from build123d import *

# Parameters (mm, degrees)
BOSS_EXTRUDE1_DEPTH     = 40
SKETCH2_R               = 2.6
CUT_EXTRUDE1_DEPTH      = 40
CUT_EXTRUDE2_DEPTH      = 3
CUT_EXTRUDE3_DEPTH      = 52.23475383
CUT_EXTRUDE3_DEPTH_BACK = 52.23475383
SKETCH4_R               = 2.6
CUT_EXTRUDE4_DEPTH      = 3
CHAMFER1_SIZE           = 10


with BuildPart() as part:
    # Sketch1 → Boss-Extrude1 (new body)
    with BuildSketch(Plane(origin=(0, 0, 0), x_dir=(1, 0, 0), z_dir=(0, 1, 0))):
        Polygon((0, 0), (25, 0), (25, 5), (5, 5), (5, 25), (0, 25), align=None)
    extrude(amount=BOSS_EXTRUDE1_DEPTH)

    # Sketch2 → Cut-Extrude1 (cut)
    with BuildSketch(Plane(origin=(0, 0, -5), x_dir=(-1, 0, 0), z_dir=(0, 0, -1))):
        with Locations((-17, 20)):
            Circle(SKETCH2_R)
    extrude(amount=-CUT_EXTRUDE1_DEPTH, mode=Mode.SUBTRACT)

    # Sketch3 → Cut-Extrude2 (cut)
    with BuildSketch(Plane(origin=(0, 0, -5), x_dir=(-1, 0, 0), z_dir=(0, 0, -1))):
        Polygon((-14.546261356, 24.25), (-19.453738644, 24.25), (-21.907477288, 20), (-19.453738644, 15.75), (-14.546261356, 15.75), (-12.092522712, 20), align=None)
    extrude(amount=-CUT_EXTRUDE2_DEPTH, mode=Mode.SUBTRACT)

    # Sketch4 → Cut-Extrude3 (cut, two sides: drawn at the far end of the back side and taken through both)
    with BuildSketch(Plane(origin=(5, 0, 0), x_dir=(0, 0, -1), z_dir=(1, 0, 0)).offset(-CUT_EXTRUDE3_DEPTH_BACK)):
        with Locations((17, 20)):
            Circle(SKETCH4_R)
    extrude(amount=CUT_EXTRUDE3_DEPTH + CUT_EXTRUDE3_DEPTH_BACK, mode=Mode.SUBTRACT)

    # Sketch5 → Cut-Extrude4 (cut)
    with BuildSketch(Plane(origin=(5, 0, 0), x_dir=(0, 0, -1), z_dir=(1, 0, 0))):
        Polygon((19.453738644, 24.25), (14.546261356, 24.25), (12.092522712, 20), (14.546261356, 15.75), (19.453738644, 15.75), (21.907477288, 20), align=None)
    extrude(amount=-CUT_EXTRUDE4_DEPTH, mode=Mode.SUBTRACT)

    # Chamfer1
    chamfer1_edges = [part.edges().sort_by_distance(p)[0] for p in [
        (25, 40, -2.5),
        (2.5, 40, -25),
        (2.5, 0, -25),
        (25, 0, -2.5),
    ]]
    chamfer(chamfer1_edges, length=CHAMFER1_SIZE)


solid = part.part
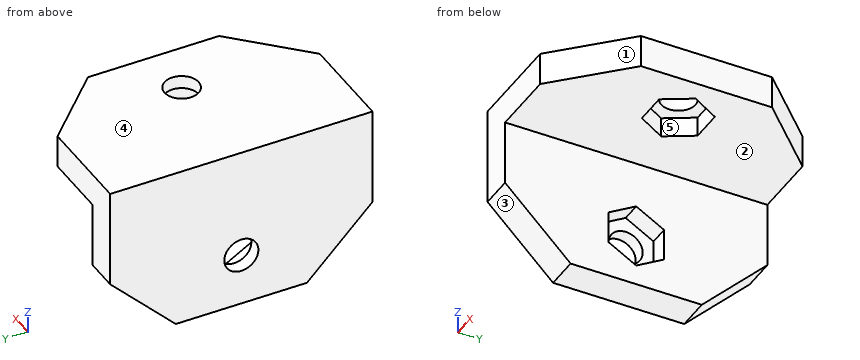
Verification items for the finished model (mm, model axes). Face numbers are marked on the shaded views. A direction names the side the tool comes from. Coordinates: 2 decimals unless noted, no trailing zeros. Order: outer loops, then holes, each group sorted by start corner. A loop starts at its lowest first (then second) coordinate and runs counter-clockwise, first axis right, second up. Notation, with made-up numbers: (87, -18.5) -> (141, -18.5) arc R18 ccw to (141, -8.5) -> close; hole circle Ø4 at (-10, -32.5). An arc over 180 degrees is marked (long way). Put each result on its own line as item: value. Start each with the question number.
1. Mould release check, pull along Y, two halves, no side actions. Record for the marked faces 3, 4 and 5: released by +Y, released by -Y, zero draft, split by the parting line, or undercut.
2. Access from +Z, -Z, +X, -X, +Y, -Y to the whole of each face (thin tool, end or side, straight path). Record for the marked faces 1 and 2.
3. Cross-section at A-A, the plane x = 17. Record the boundary of the cut face in (y, z), then the cut area to 3 significant figures.
4. Cross-section at D-D, the plane z = -13.75. Record the boundary of the cut face in (x, y), then the cut area to 3 significant figures.
5. Cross-section at C-C, the plane y = 18.5. Record the boundary of the cut face in (x, z).
6. Cross-section at B-B, the plane z = -17. Record the boundary of the cut face in (x, y).
7. Go/stop test with flat-tipped pins: pin 1 Ø12 at (x, z) = (13, -11.5) entering from -Y; pin 2 Ø3 at (x, y) = (10.5, 7) entering from -Z; pin 3 Ø2.5 at (x, z) = (4, -18) entering from +Y; pin 4 Ø2.5 at (x, z) = (16.5, -3) entering from -Y. Record where each tip stops, or that it passes through.
8. Material ranges on L1, parallel to Z at x = 1, y = 20; L2, parallel to Y at x = 2.5, z = -14.75; L3, parallel to X at y = 9, z = -10.25, recorded low to high. Write a range as [from, to].
Computed:
1. face 3: released by -Y
1. face 4: zero draft
1. face 5: undercut
2. face 1: +Z, -Z, +X, -Y
2. face 2: -Z, +X, +Y, -Y
3. outline: (2, -5) -> (15.75, -5) -> (15.75, -2) -> (17.4, -2) -> (17.4, 0) -> (2, 0) -> close; (22.6, -2) -> (24.25, -2) -> (24.25, -5) -> (38, -5) -> (38, 0) -> (22.6, 0) -> close
3. area: 144 mm2
4. outline: (0, 0) -> (5, 0) -> (5, 17.13) -> (2, 17.13) -> (2, 22.87) -> (5, 22.87) -> (5, 40) -> (0, 40) -> close
4. area: 183 mm2
5. outline: (0, -25) -> (5, -25) -> (5, -21.04) -> (2, -21.04) -> (2, -19.12) -> (0, -19.12) -> close; (0, -14.88) -> (2, -14.88) -> (2, -12.96) -> (5, -12.96) -> (5, -5) -> (12.96, -5) -> (12.96, -2) -> (14.88, -2) -> (14.88, 0) -> (0, 0) -> close; (19.12, -2) -> (21.04, -2) -> (21.04, -5) -> (25, -5) -> (25, 0) -> (19.12, 0) -> close
6. outline: (0, 2) -> (5, 2) -> (5, 15.75) -> (2, 15.75) -> (2, 17.4) -> (0, 17.4) -> close; (0, 22.6) -> (2, 22.6) -> (2, 24.25) -> (5, 24.25) -> (5, 38) -> (0, 38) -> close
7. pin 1: through
7. pin 2: z = -5
7. pin 3: y = 38.25
7. pin 4: y = 0.25
8. L1: [-25, -19.6], [-14.4, 0]
8. L2: [0, 15.75], [24.25, 40]
8. L3: [0, 5]
